Geometry: final body of the model. Coordinates: model frame, mm. A direction names the side the tool comes from. Give positions to 0.01 mm unless a question says otherwise; leave off trailing zeros. Write each loop counter-clockwise with the first axis right and the second up, starting at its lowest first coordinate (ties: lowest second). Pieces come first, ordered by that corner, then holes.
Autodesk Inventor part; units mm, degrees
ref_plane "YZ Plane" through (0, 0, 0) normal (1, 0, 0) x (0, 1, 0)
ref_plane "XZ Plane" through (0, 0, 0) normal (0, 1, 0) x (-1, 0, 0)
ref_plane "XY Plane" through (0, 0, 0) normal (0, 0, 1) x (1, 0, 0)
sketch "草图1" plane through (0, 0, 0) normal (0, 1, 0) x (-1, 0, 0)
  line L0 (-40, 80) -> (40, 80)
  line L1 (40, 80) -> (40, -80)
  line L2 (40, -80) -> (-40, -80)
  line L3 (-40, -80) -> (-40, 80)
  line L4 (-40, 80) -> (40, -80) construction
  line L5 (40, 80) -> (-40, -80) construction
  point P0 (0, 0)
  dimension "d0" = 160
  dimension "d1" = 80
extrude "拉伸1" add sketch "草图1" along normal blind 15
sketch "草图2" plane through (0, 15, 0) normal (0, 1, 0) x (1, 0, 0)
  line L0 (25, -45) -> (-25, -45)
  line L1 (-25, -45) -> (-25, 45)
  line L2 (-25, 45) -> (25, 45)
  line L3 (25, 45) -> (25, -45)
  line L4 (25, -45) -> (-25, 45) construction
  line L5 (-25, -45) -> (25, 45) construction
  point P0 (0, 0)
  dimension "d4" = 90
  dimension "d5" = 50
extrude "拉伸2" add sketch "草图2" along normal blind 30
sketch "草图3" plane through (0, 0, 0) normal (1, 0, 0) x (0, 1, 0)
  line L0 (0, 0) -> (70, 0) construction
  arc A0 (70, -20) -> (70, 20) centre (70, 0) ccw
  line L1 (70, 20) -> (15, 20)
  line L2 (15, -80) -> (15, 80) construction
  line L3 (70, -20) -> (15, -20)
  line L4 (15, -20) -> (15, 20)
  circle A1 centre (70, 0) radius 10
  line L5 (0, 80) -> (0, -80)
  dimension "d8" = 20
  dimension "d9" = 20
  dimension "d10" = 70
extrude "拉伸3" add sketch "草图3" along normal mid plane 60
sketch "草图4" plane through (0, 15, 0) normal (0, 1, 0) x (1, 0, 0)
  line L0 (25, -65) -> (-25, -65) construction
  line L1 (-25, -65) -> (-25, 65) construction
  line L2 (-25, 65) -> (25, 65) construction
  line L3 (25, 65) -> (25, -65) construction
  line L4 (25, -65) -> (-25, 65) construction
  line L5 (-25, -65) -> (25, 65) construction
  circle A0 centre (-25, -65) radius 7.5
  circle A1 centre (-25, 65) radius 7.5
  circle A2 centre (25, 65) radius 7.5
  circle A3 centre (25, -65) radius 7.5
  point P0 (0, 0)
  dimension "d13" = 130
  dimension "d14" = 50
  dimension "d15" = 15
extrude "拉伸4" cut sketch "草图4" against normal blind 60
fillet "圆角1" radius 15 4 edges at (40, 7.5, 80) (40, 7.5, -80) (-40, 7.5, 80) (-40, 7.5, -80)
fillet "圆角2" radius 20 2 edges at (-25, 30, -45) (-25, 30, 45)
sketch "草图5" plane through (0, 0, 0) normal (0, 1, 0) x (-1, 0, 0)
  line L0 (0, 0) -> (-35, 0) construction
  arc A0 (-35, -40) -> (-35, 40) centre (-35, 0) ccw
  line L1 (-40, 65) -> (-40, -65) construction
  line L2 (-35, 40) -> (-40, 40)
  line L3 (-40, 40) -> (-40, -40)
  line L4 (-40, -40) -> (-35, -40)
  dimension "d20" = 5
  dimension "d21" = 40
extrude "拉伸5" cut sketch "草图5" along normal blind 35
sketch "草图6" plane through (0, 0, 0) normal (1, 0, 0) x (0, 1, 0)
  arc A0 (70, -20) -> (70, 20) centre (70, 0) ccw
  line L0 (70, 20) -> (35, 20)
  line L1 (45, 45) -> (45, 20)
  line L2 (15, 45) -> (45, 45)
  line L3 (15, 65) -> (15, 40)
  line L4 (15, 80) -> (15, 65)
  line L5 (15, 80) -> (83.7931, 14.4828)
  arc A1 (70, -20) -> (70, 20) centre (70, 0) ccw
  arc A2 (83.7931, 14.4828) -> (70, 20) centre (70, 0) ccw
  line L6 (45, 20) -> (45, 25)
  line L7 (70, 20) -> (45, 20)
  line L8 (45, 45) -> (45, 25)
  line L9 (45, 20) -> (45, 45)
  line L10 (15, 45) -> (45, 45)
  line L11 (45, 45) -> (15, 45)
  line L12 (15, 80) -> (15, 65)
  line L13 (15, 45) -> (15, 80)
  point P0 (0, 0)
extrude "拉伸6" add sketch "草图6" along normal mid plane 10
mirror "镜像1" about plane through (0, 0, 0) normal (0, 0, 1) of "拉伸6"
properties part number "模型2"
Q1. Section C-C on x = 22.5. Output: boundary loops of the cut face in (y, z).
Filled sheet:
outline: (0, -80) - (15, -80) - (15, -72.07) - (0, -72.07) - close; (0, -57.93) - (15, -57.93) - (15, -45) - (45, -45) - (45, -20) - (70, -20) arc R20 ccw to (70, 20) - (45, 20) - (45, 45) - (15, 45) - (15, 57.93) - (0, 57.93) - (0, 38) - (35, 38) - (35, -38) - (0, -38) - close; (0, 72.07) - (15, 72.07) - (15, 80) - (0, 80) - close; hole circle Ø20 at (70, 0)
Q2. Section B-B on x = 11. Output: boundary loops of the cut face in (y, z), plus the area to 3 significant figures.
Filled sheet:
outline: (0, -80) - (15, -80) - (15, -45) - (45, -45) - (45, -20) - (70, -20) arc R20 ccw to (70, 20) - (45, 20) - (45, 45) - (15, 45) - (15, 80) - (0, 80) - (0, 32) - (35, 32) - (35, -32) - (0, -32) - close; hole circle Ø20 at (70, 0)
area: 4,170 mm2
Q3. Pull-direction query (Z, two-part tool) for faces 1 (the cylindrical face through (-19.297, 30.21, 38.986)), 2 (the flat face through (13, 35, 1)), 3 (the flat face through (15, 30, -45)), 4 (the flat face through (-30, 44, 0)); classes: released by +Z, released by -Z, zero draft, split by the parting line, or undercut.
Filled sheet:
face 1: released by +Z
face 2: undercut
face 3: released by -Z
face 4: zero draft
Q4. Ray query, line 1 along X through (y, z) = (11, -65); line 2 along Z through (x, y) = (25, 4); line 3 along Z through (x, y) = (-25, 11). Return the intervals inside material, ascending.
Filled sheet:
line 1: x = -40 to -32.5, -17.5 to 17.5, 32.5 to 40
line 2: z = -80 to -72.5, -57.5 to -38.73, 38.73 to 57.5, 72.5 to 80
line 3: z = -80 to -72.5, -57.5 to 57.5, 72.5 to 80
Q5. Pin query (flat end, axial travel): P1, Ø1.5, axis at x = 36.5, y = 11, coming from the +Z side; P2, Ø3, axis at x = -27.5, y = 12.5, coming from the -Z side; P3, Ø1, axis at y = 31.5, z = -56, coming from the +X side; P4, Ø12, axis at y = 70, z = 0, coming from the -X side. Return the tip coordinate at first contact, or that it passes through.
Filled sheet:
P1: stops at z = 75.46
P2: stops at z = -79.97
P3: stops at x = 5
P4: passes through
Q6. Section A-A on z = 0. Output: boundary loops of the cut face in (x, y).
Filled sheet:
outline: (-40, 0) - (-5, 0) - (-5, 35) - (30, 35) - (30, 60) - (-30, 60) - (-30, 15) - (-40, 15) - close; (-30, 80) - (30, 80) - (30, 90) - (-30, 90) - close
Q7. Access query for faces 5 (the cylindrical face through (0, 90, 0)), 6 (the flat face through (15, 45, 32)), 7 (the flat face through (-25, 30, -22)). Directions: +Z, -Z, +X, -X, +Y, -Y. A direction counts if a zero-diameter tool reaches every point of the face in a straight line with its end or side. Return the directions, or none.
Filled sheet:
face 5: +Y
face 6: +Z, +X, +Y
face 7: -Z, -X, +Y
Q8. Section D-D on y = 63. Output: boundary loops of the cut face in (x, z), plus the area to 3 significant figures.
Filled sheet:
outline: (-30, -20) - (-5, -20) - (-5, -34.29) - (5, -34.29) - (5, -20) - (30, -20) - (30, -7.14) - (-30, -7.14) - close; (-30, 7.14) - (30, 7.14) - (30, 20) - (5, 20) - (5, 34.29) - (-5, 34.29) - (-5, 20) - (-30, 20) - close
area: 1,830 mm2
